Verification items for the finished model (mm, model axes). Coordinates: 2 decimals unless noted, no trailing zeros. Order: outer loops, then holes, each group sorted by start corner. A loop starts at its lowest first (then second) coordinate and runs counter-clockwise, first axis right, second up. Notation, with made-up numbers: (-9, -38.75) - (-3, -38.75) arc R22 cw to (-3, -11.75) - close; hole circle Ø6 at (11, 83). An arc over 180 degrees is marked (long way). Answer as CSV lines item,"result". Start each with the question number.
1. Go/stop test with flat-tipped pins: pin 1 (2.5 mm diameter, centred on x = 33.39, z = -124.6, fed in from +Y); pin 2 (2 mm diameter, centred on x = -32.5, z = -125.5, fed in from +Y); pin 3 (1 mm diameter, centred on y = 1, z = 17.5, fed in from +X); pin 4 (1 mm diameter, centred on y = 3, z = -72, fed in from -X). Record where each tip stops, or that it passes through.
2. Section check C-C (y = 2.6). Count the separate pieces of the cut face and the enclosed holes in it, and give its area (3 significant figures).
3. Section check A-A (z = 0). Record the cut outline in (x, y), and give its area (3 significant figures).
4. Material ranges on L1, parallel to Z at x = 0, y = 1.2; L2, parallel to Z at x = 127, y = 3.1; L3, parallel to Z at x = 91.5, y = 3.4, recorded low to high. Write a range as [from, to].
5. Section check B-B (x = 0). Record the cut outline in (y, z), and give its area (3 significant figures).
Autodesk Inventor part; units mm, degrees
ref_plane "YZ Plane" through (0, 0, 0) normal (1, 0, 0) x (0, 1, 0)
ref_plane "XZ Plane" through (0, 0, 0) normal (0, 1, 0) x (-1, 0, 0)
ref_plane "XY Plane" through (0, 0, 0) normal (0, 0, 1) x (1, 0, 0)
sketch "Sketch1" plane through (0, 0, 0) normal (0, 1, 0) x (-1, 0, 0)
  circle A0 centre (0, 0) radius 150
  circle A1 centre (0, 0) radius 125
  dimension "d0" = 300
  dimension "d1" = 250
extrude "Extrusion1" add sketch "Sketch1" along normal blind 4
sketch "Sketch2" plane through (0, 4, 0) normal (0, 1, 0) x (1, 0, 0)
  line L0 (0, 0) -> (124.6044, 33.3877) construction
  line L1 (125.4861, 30.0974) -> (122.1958, 30.979)
  line L2 (122.1958, 30.979) -> (121.3141, 34.2693)
  line L3 (121.3141, 34.2693) -> (123.7228, 36.678)
  line L4 (123.7228, 36.678) -> (127.0131, 35.7963)
  line L5 (127.0131, 35.7963) -> (127.8947, 32.506)
  line L6 (127.8947, 32.506) -> (125.4861, 30.0974)
  line L7 (0, 0) -> (150, 0) construction
  circle A0 centre (0, 0) radius 150
  line L8 (87.9265, 90.3351) -> (88.8081, 93.6254)
  line L9 (90.3351, 87.9265) -> (87.9265, 90.3351)
  line L10 (93.6254, 88.8081) -> (90.3351, 87.9265)
  line L11 (94.5071, 92.0984) -> (93.6254, 88.8081)
  line L12 (92.0984, 94.5071) -> (94.5071, 92.0984)
  line L13 (88.8081, 93.6254) -> (92.0984, 94.5071)
  line L14 (30.979, 122.1958) -> (30.0974, 125.4861)
  line L15 (34.2693, 121.3141) -> (30.979, 122.1958)
  line L16 (36.678, 123.7228) -> (34.2693, 121.3141)
  line L17 (35.7963, 127.0131) -> (36.678, 123.7228)
  line L18 (32.506, 127.8947) -> (35.7963, 127.0131)
  line L19 (30.0974, 125.4861) -> (32.506, 127.8947)
  line L20 (-34.2693, 121.3141) -> (-36.678, 123.7228)
  line L21 (-30.979, 122.1958) -> (-34.2693, 121.3141)
  line L22 (-30.0974, 125.4861) -> (-30.979, 122.1958)
  line L23 (-32.506, 127.8947) -> (-30.0974, 125.4861)
  line L24 (-35.7963, 127.0131) -> (-32.506, 127.8947)
  line L25 (-36.678, 123.7228) -> (-35.7963, 127.0131)
  line L26 (-90.3351, 87.9265) -> (-93.6254, 88.8081)
  line L27 (-87.9265, 90.3351) -> (-90.3351, 87.9265)
  line L28 (-88.8081, 93.6254) -> (-87.9265, 90.3351)
  line L29 (-92.0984, 94.5071) -> (-88.8081, 93.6254)
  line L30 (-94.5071, 92.0984) -> (-92.0984, 94.5071)
  line L31 (-93.6254, 88.8081) -> (-94.5071, 92.0984)
  line L32 (-122.1958, 30.979) -> (-125.4861, 30.0974)
  line L33 (-121.3141, 34.2693) -> (-122.1958, 30.979)
  line L34 (-123.7228, 36.678) -> (-121.3141, 34.2693)
  line L35 (-127.0131, 35.7963) -> (-123.7228, 36.678)
  line L36 (-127.8947, 32.506) -> (-127.0131, 35.7963)
  line L37 (-125.4861, 30.0974) -> (-127.8947, 32.506)
  line L38 (-121.3141, -34.2693) -> (-123.7228, -36.678)
  line L39 (-122.1958, -30.979) -> (-121.3141, -34.2693)
  line L40 (-125.4861, -30.0974) -> (-122.1958, -30.979)
  line L41 (-127.8947, -32.506) -> (-125.4861, -30.0974)
  line L42 (-127.0131, -35.7963) -> (-127.8947, -32.506)
  line L43 (-123.7228, -36.678) -> (-127.0131, -35.7963)
  line L44 (-87.9265, -90.3351) -> (-88.8081, -93.6254)
  line L45 (-90.3351, -87.9265) -> (-87.9265, -90.3351)
  line L46 (-93.6254, -88.8081) -> (-90.3351, -87.9265)
  line L47 (-94.5071, -92.0984) -> (-93.6254, -88.8081)
  line L48 (-92.0984, -94.5071) -> (-94.5071, -92.0984)
  line L49 (-88.8081, -93.6254) -> (-92.0984, -94.5071)
  line L50 (-30.979, -122.1958) -> (-30.0974, -125.4861)
  line L51 (-34.2693, -121.3141) -> (-30.979, -122.1958)
  line L52 (-36.678, -123.7228) -> (-34.2693, -121.3141)
  line L53 (-35.7963, -127.0131) -> (-36.678, -123.7228)
  line L54 (-32.506, -127.8947) -> (-35.7963, -127.0131)
  line L55 (-30.0974, -125.4861) -> (-32.506, -127.8947)
  line L56 (34.2693, -121.3141) -> (36.678, -123.7228)
  line L57 (30.979, -122.1958) -> (34.2693, -121.3141)
  line L58 (30.0974, -125.4861) -> (30.979, -122.1958)
  line L59 (32.506, -127.8947) -> (30.0974, -125.4861)
  line L60 (35.7963, -127.0131) -> (32.506, -127.8947)
  line L61 (36.678, -123.7228) -> (35.7963, -127.0131)
  line L62 (90.3351, -87.9265) -> (93.6254, -88.8081)
  line L63 (87.9265, -90.3351) -> (90.3351, -87.9265)
  line L64 (88.8081, -93.6254) -> (87.9265, -90.3351)
  line L65 (92.0984, -94.5071) -> (88.8081, -93.6254)
  line L66 (94.5071, -92.0984) -> (92.0984, -94.5071)
  line L67 (93.6254, -88.8081) -> (94.5071, -92.0984)
  line L68 (122.1958, -30.979) -> (125.4861, -30.0974)
  line L69 (121.3141, -34.2693) -> (122.1958, -30.979)
  line L70 (123.7228, -36.678) -> (121.3141, -34.2693)
  line L71 (127.0131, -35.7963) -> (123.7228, -36.678)
  line L72 (127.8947, -32.506) -> (127.0131, -35.7963)
  line L73 (125.4861, -30.0974) -> (127.8947, -32.506)
  dimension "d4" = 5.9
  dimension "d5" = 15
  dimension "d6" = 129
  dimension "d9" = 360
extrude "Extrusion2" cut sketch "Sketch2" against normal blind 2 contours L1 L2 L3 L4 L5 L6 | L8 L13 L12 L11 L10 L9 | L14 L19 L18 L17 L16 L15 | L20 L25 L24 L23 L22 L21 | L26 L31 L30 L29 L28 L27 | L32 L37 L36 L35 L34 L33 | L38 L43 L42 L41 L40 L39 | L44 L49 L48 L47 L46 L45 | L50 L55 L54 L53 L52 L51 | L56 L61 L60 L59 L58 L57 | L62 L67 L66 L65 L64 L63 | L68 L73 L72 L71 L70 L69
sketch "Sketch3" plane through (0, 2, 0) normal (0, 1, 0) x (1, 0, 0)
  line L0 (121.3141, 34.2693) -> (123.7228, 36.678)
  line L1 (125.4861, 30.0974) -> (122.1958, 30.979)
  line L2 (123.7228, 36.678) -> (125.4861, 30.0974) construction
  circle A0 centre (124.6044, 33.3877) radius 1.7
  circle A1 centre (91.2168, 91.2168) radius 1.7
  circle A2 centre (33.3877, 124.6044) radius 1.7
  circle A3 centre (-33.3877, 124.6044) radius 1.7
  circle A4 centre (-91.2168, 91.2168) radius 1.7
  circle A5 centre (-124.6044, 33.3877) radius 1.7
  circle A6 centre (-124.6044, -33.3877) radius 1.7
  circle A7 centre (-91.2168, -91.2168) radius 1.7
  circle A8 centre (-33.3877, -124.6044) radius 1.7
  circle A9 centre (33.3877, -124.6044) radius 1.7
  circle A10 centre (91.2168, -91.2168) radius 1.7
  circle A11 centre (124.6044, -33.3877) radius 1.7
  point P0 (0, 0)
  dimension "d13" = 3.4
  dimension "d16" = 360
extrude "Extrusion3" cut sketch "Sketch3" against normal through all
properties part number "ArmLoopInnerRing"
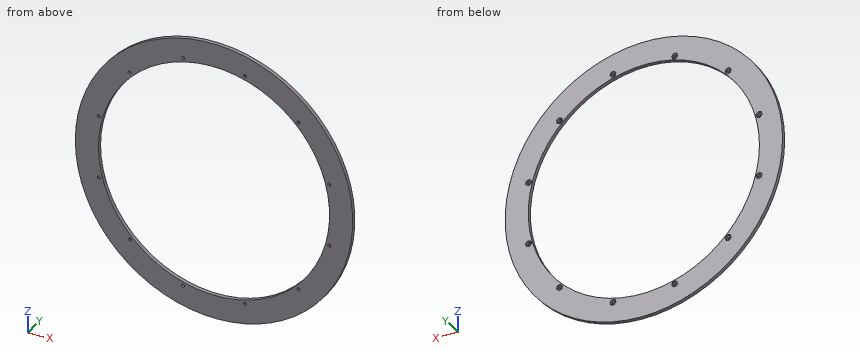
Evaluation:
1,pin 1,"passes through"
1,pin 2,"stops at y = 2"
1,pin 3,"stops at x = 149.03"
1,pin 4,"stops at x = -131.86"
2,separate pieces,"1"
2,enclosed holes,"13"
2,area,"21,200 mm²"
3,outline,"(-150, 0) - (-125, 0) - (-125, 4) - (-150, 4) - close; (125, 0) - (150, 0) - (150, 4) - (125, 4) - close"
3,area,"200 mm²"
4,L1,"z = [-150, -125], [125, 150]"
4,L2,"z = [-79.82, -35.8], [-31.61, 31.61], [35.8, 79.82]"
4,L3,"z = [-118.86, -94.35], [-88.24, -85.16], [85.16, 88.24], [94.35, 118.86]"
5,outline,"(0, -150) - (4, -150) - (4, -125) - (0, -125) - close; (0, 125) - (4, 125) - (4, 150) - (0, 150) - close"
5,area,"200 mm²"
